Geometry: final body of the model. Coordinates: model frame, mm. A direction names the side the tool comes from. Give positions to 0.01 mm unless a question says otherwise; leave off trailing zeros. Order: outer loops, then holes, each group sorted by start corner. A loop starts at its lowest first (then second) coordinate and runs counter-clockwise, first axis right, second up. Notation, with made-up numbers: (59.5, -2.5) - (114.5, -2.5) arc R16 ccw to (114.5, 20.5) - close; hole circle Ø4 at (-25.75, 23.25). An arc over 180 degrees is marked (long way). One line per item, written item: value.
```python
from build123d import *

# Parameters (mm, degrees)
SKETCH1_R           = 47.5
BOSS_EXTRUDE1_DEPTH = 4
SKETCH2_R           = 22.5
CUT_EXTRUDE1_DEPTH  = 68.294130502
SKETCH3_R           = 4.231561453
CUT_EXTRUDE2_DEPTH  = 4
CIRPATTERN1_DEPTH   = 4


# Read off the part's stored shape, not the designer's step: CirPattern1
with BuildPart() as part:
    # Sketch1 → Boss-Extrude1 (new body)
    with BuildSketch(Plane(origin=(0, 0, 0), x_dir=(1, 0, 0), z_dir=(0, 1, 0))):
        with Locations(Location((0, 0, 0), (0, 0, 270))):
            Circle(SKETCH1_R)
    extrude(amount=BOSS_EXTRUDE1_DEPTH)

    # Sketch2 → Cut-Extrude1 (cut, through all)
    with BuildSketch(Plane(origin=(0, 0, 0), x_dir=(1, 0, 0), z_dir=(0, 1, 0))):
        with Locations(Location((0, 0, 0), (0, 0, 270))):
            Circle(SKETCH2_R)
    extrude(amount=CUT_EXTRUDE1_DEPTH, mode=Mode.SUBTRACT)

    # Sketch3 → Cut-Extrude2 (cut)
    with BuildSketch(Plane(origin=(0, 4, 0), x_dir=(1, 0, 0), z_dir=(0, 1, 0))):
        with Locations((-19.192330033, 0)):
            Circle(SKETCH3_R)
    extrude(amount=-CUT_EXTRUDE2_DEPTH, mode=Mode.SUBTRACT)

    # CirPattern1 outline → CirPattern1 (cut)
    with BuildSketch(Plane(origin=(0, 0, 0), x_dir=(1, 0, 0), z_dir=(0, 1, 0))):
        with BuildLine():
            ThreePointArc((-13.765038141, -17.798138245), (-15.909902577, -15.909902577), (-17.798138245, -13.765038141))
            ThreePointArc((-17.798138245, -13.765038141), (-16.563192512, -16.563192512), (-13.765038141, -17.798138245))
        make_face()
        with BuildLine():
            ThreePointArc((-17.798138245, 13.765038141), (-15.909902577, 15.909902577), (-13.765038141, 17.798138245))
            ThreePointArc((-13.765038141, 17.798138245), (-16.563192512, 16.563192512), (-17.798138245, 13.765038141))
        make_face()
        with BuildLine():
            ThreePointArc((-2.851832433, 22.318536059), (0, 22.500000001), (2.851832433, 22.318536059))
            ThreePointArc((2.851832433, 22.318536059), (0, 23.423891487), (-2.851832433, 22.318536059))
        make_face()
        with BuildLine():
            ThreePointArc((13.765038141, 17.798138245), (15.909902577, 15.909902577), (17.798138245, 13.765038141))
            ThreePointArc((17.798138245, 13.765038141), (16.563192512, 16.563192512), (13.765038141, 17.798138245))
        make_face()
        with BuildLine():
            ThreePointArc((22.318536058, 2.851832433), (22.5, 0), (22.318536058, -2.851832433))
            ThreePointArc((22.318536058, -2.851832433), (23.423891487, 0), (22.318536058, 2.851832433))
        make_face()
        with BuildLine():
            ThreePointArc((17.798138245, -13.765038141), (15.909902576, -15.909902576), (13.765038141, -17.798138244))
            ThreePointArc((13.765038141, -17.798138244), (16.563192512, -16.563192512), (17.798138245, -13.765038141))
        make_face()
        with BuildLine():
            ThreePointArc((2.851832433, -22.318536058), (0, -22.499999999), (-2.851832433, -22.318536058))
            ThreePointArc((-2.851832433, -22.318536058), (0, -23.423891487), (2.851832433, -22.318536058))
        make_face()
    extrude(amount=CIRPATTERN1_DEPTH, mode=Mode.SUBTRACT)


solid = part.part
```
1) Section B-B, the plane z = 0. Return loops of the section in (x, y).
Answers below:
outline: (-47.5, 0) - (-23.42, 0) - (-23.42, 4) - (-47.5, 4) - close; (23.42, 0) - (47.5, 0) - (47.5, 4) - (23.42, 4) - close
2) Mould query, pull axis X, two halves, no side actions, for faces 1 (the face through (-9.9, 0, 20.4)), 2 (the face through (20.82, 1.97, -8.53)), 3 (the face through (-46.37, 1.97, -10.3)). Classes: released by +X, released by -X, zero draft, split by the parting line, or undercut.
Answers below:
face 1: zero draft
face 2: undercut
face 3: split by the parting line
3) Section A-A, the plane x = 0. Return loops of the section in (y, z), then the cut area to 3 significant figures.
Answers below:
outline: (0, -47.5) - (4, -47.5) - (4, -23.42) - (0, -23.42) - close; (0, 23.42) - (4, 23.42) - (4, 47.5) - (0, 47.5) - close
area: 193 mm^2
4) Set-up query: faces 4 (the face through (-9.9, 4, 20.4)), 5 (the face through (16.594, 1.972, -16.532)). Return all of +Z, -Z, +X, -X, +Y, -Y with unobstructed straight access to the full face (end or side cutting, diameter ignored); none if empty.
Answers below:
face 4: +Z, -Z, +X, -X, +Y
face 5: +Y, -Y
5) Section D-D, the plane x = 33. Return loops of the section in (y, z), then the cut area to 3 significant figures.
Answers below:
outline: (0, -34.17) - (4, -34.17) - (4, 34.17) - (0, 34.17) - close
area: 273 mm^2
6) First-contact query: pin 1 (1.5 mm diameter, centred on y = 1, z = 15.5, fed in from +X); pin 2 (1.5 mm diameter, centred on y = 3, z = 16.5, fed in from +X). Flat tips, straight axial feed; report the tip coordinate or a pass-through.
Answers below:
pin 1: x = 45.15
pin 2: x = 44.81
7) Material intervals for line 1 along X through (y, z) = (1.9, 10); line 2 along X through (y, z) = (3.15, 14.5); line 3 along Z through (x, y) = (-19, 3.5), sorted ascending.
Answers below:
line 1: -46.44 to -20.16, 20.16 to 46.44
line 2: -45.23 to -17.7, 17.7 to 45.23
line 3: -43.53 to -12.05, 12.05 to 43.53
8) Section C-C, the plane y = 2.8. Return loops of the section in (x, z).
Answers below:
outline: circle Ø95 at (0, 0); hole (-22.32, -2.85) arc R22.5 ccw to (-17.8, -13.77) arc R4.23 ccw to (-13.77, -17.8) arc R22.5 ccw to (-2.85, -22.32) arc R4.23 ccw to (2.85, -22.32) arc R22.5 ccw to (13.77, -17.8) arc R4.23 ccw to (17.8, -13.77) arc R22.5 ccw to (22.32, -2.85) arc R4.23 ccw to (22.32, 2.85) arc R22.5 ccw to (17.8, 13.77) arc R4.23 ccw to (13.77, 17.8) arc R22.5 ccw to (2.85, 22.32) arc R4.23 ccw to (-2.85, 22.32) arc R22.5 ccw to (-13.77, 17.8) arc R4.23 ccw to (-17.8, 13.77) arc R22.5 ccw to (-22.32, 2.85) arc R4.23 ccw to start
